Autodesk Fusion 360 part; units mm, degrees
sketch "Sketch1" plane through (0, 0, 0) normal (0, 0, 1) x (1, 0, 0)
  line L0 (0, 0) -> (50.8, 0)
  line L1 (50.8, 0) -> (50.8, 50.8)
  line L2 (50.8, 50.8) -> (0, 50.8)
  line L3 (0, 50.8) -> (0, 0)
  dimension "d1" = 50.8
  dimension "d2" = 50.8
extrude "Extrude1" add sketch "Sketch1" along normal blind 31.75
sketch "Sketch2" plane through (50.8, 0, 0) normal (1, 0, 0) x (0, 1, 0)
  line L0 (0, 0) -> (50.8, 0)
  line L1 (50.8, 0) -> (50.8, 31.75)
  line L2 (50.8, 31.75) -> (0, 31.75)
  line L3 (0, 31.75) -> (0, 0)
  line L4 (50.8, 23.368) -> (10.16, 23.368)
  line L5 (10.16, 23.368) -> (10.16, 3.81)
  line L6 (10.16, 3.81) -> (50.8, 3.81)
  line L7 (50.8, 3.81) -> (50.8, 23.368)
  dimension "d5" = 40.64
  dimension "d6" = 19.558
  dimension "d14" = 3.81
extrude "Extrude2" cut sketch "Sketch2" against normal blind 40.64 contours L1 L4 L5 L6 L7
sketch "Sketch3" plane through (0, 0, 31.75) normal (0, 0, 1) x (-1, 0, 0)
  line L0 (0, -50.8) -> (0, 0)
  line L1 (0, 0) -> (-50.8, 0)
  line L2 (-50.8, 0) -> (-50.8, -50.8)
  line L3 (-50.8, -50.8) -> (0, -50.8)
  line L4 (0, 0) -> (-25.4, 0)
  line L5 (-25.4, 0) -> (-25.4, -25.4)
  line L6 (-25.4, -25.4) -> (0, -25.4)
  line L7 (0, -25.4) -> (0, 0)
  dimension "d10" = 25.4
  dimension "d11" = 25.4
extrude "Extrude3" add sketch "Sketch3" along normal blind 152.4 contours L0 L1 L4 L5 L6 L7
fillet "Fillet1" radius 2.54 2 edges at (25.4, 12.7, 31.75) (12.7, 25.4, 31.75)
sketch "Sketch4" plane through (0, 0, 0) normal (0, 0, -1) x (1, 0, 0)
  line L0 (0, 0) -> (0, -50.8)
  line L1 (0, -50.8) -> (50.8, -50.8)
  line L2 (50.8, -50.8) -> (50.8, 0)
  line L3 (50.8, 0) -> (0, 0)
  line L4 (2.54, -2.54) -> (22.86, -2.54)
  line L5 (22.86, -2.54) -> (22.86, -22.86)
  line L6 (22.86, -22.86) -> (2.54, -22.86)
  line L7 (2.54, -22.86) -> (2.54, -2.54)
  dimension "d17" = 2.54
  dimension "d18" = 2.54
  dimension "d19" = 20.32
  dimension "d20" = 20.32
sketch "Sketch5" plane through (0, 0, 0) normal (0, 0, -1) x (1, 0, 0)
  line L0 (5.08, -5.08) -> (20.32, -5.08)
  line L1 (20.32, -5.08) -> (20.32, -20.32)
  line L2 (20.32, -20.32) -> (5.08, -20.32)
  line L3 (5.08, -20.32) -> (5.08, -5.08)
  line L4 (2.54, -2.54) -> (22.86, -2.54)
  line L5 (2.54, -22.86) -> (2.54, -2.54)
  dimension "d21" = 2.54
  dimension "d22" = 2.54
  dimension "d23" = 15.24
  dimension "d24" = 15.24
extrude "Extrude4" add sketch "Sketch5" along normal blind 2.54
loft "Loft1" add profiles "Sketch4" section 1 contours L4 L5 L6 L7 section 2 face at (10.16, 15.24, -2.54)
sketch "Sketch6" plane through (0, 0, 184.15) normal (0, 0, 1) x (-1, 0, 0)
  line L0 (0, -25.4) -> (0, 0)
  line L1 (0, 0) -> (-25.4, 0)
  line L2 (-25.4, 0) -> (-25.4, -25.4)
  line L3 (-25.4, -25.4) -> (0, -25.4)
  line L4 (-2.54, -22.86) -> (-22.86, -22.86)
  line L5 (-22.86, -22.86) -> (-22.86, -2.54)
  line L6 (-22.86, -2.54) -> (-2.54, -2.54)
  line L7 (-2.54, -2.54) -> (-2.54, -22.86)
  line L8 (-5.08, -20.32) -> (-20.32, -20.32)
  line L9 (-20.32, -20.32) -> (-20.32, -5.08)
  line L10 (-20.32, -5.08) -> (-5.08, -5.08)
  line L11 (-5.08, -5.08) -> (-5.08, -20.32)
  dimension "d27" = 2.54
  dimension "d28" = 2.54
  dimension "d29" = 2.54
  dimension "d30" = 20.32
  dimension "d31" = 2.54
  dimension "d32" = 15.24
  dimension "d33" = 15.24
  dimension "d34" = 2.54
extrude "Extrude5" cut sketch "Sketch6" against normal blind 2.54 contours L8 L9 L10 L11
loft "Loft2" cut profiles "Sketch6" section 1 contours L4 L5 L6 L7 section 2 face at (15.24, 15.24, 181.61)
Geometry: final body of the model. Coordinates: model frame, mm. A direction names the side the tool comes from. Round coordinates to 2 decimals unless told otherwise and drop trailing zeros. Order: outer loops, then holes, each group sorted by start corner. A loop starts at its lowest first (then second) coordinate and runs counter-clockwise, first axis right, second up. Notation, with made-up numbers: (38, 62) - (52, 62) arc R18 cw to (52, 84) - close; hole circle Ø7 at (88, 62.25). An arc over 180 degrees is marked (long way). Write item = value, one per line. Start each with the question number.
Q1. Cut plane A-A on y = 40.5. Return the cut outline in (x, z), and give its area (3 significant figures).
Q2. Pull-direction query (Y, two-part tool) for faces 1 (the flat face through (31, 31, 23.368)), 2 (the flat face through (13, 13, 181.61)), 3 (the flat face through (20, 50.8, 26)); classes: +Y half, -Y half, draft (parallel to the pull), parting line (faces both ways), or undercut.
Q3. Pin query (flat end, axial travel): pin 1 (3 mm diameter, centred on x = 29.5, y = 9.5, fed in from +Z); pin 2 (7.5 mm diameter, centred on x = 9, y = 14.5, fed in from +Z); pin 3 (6 mm diameter, centred on x = 24, z = 18.5, fed in from +Y). Return the tip coordinate at first contact, or that it passes through.
Q4. Ray query, line 1 (Z direction, x = 28, y = 31); line 2 (X direction, y = 25, z = 108). Return the intervals inside material, ascending. Write a range as from..to.
Q5. Cut plane C-C on z = 133. Return the cut outline in (x, y).
Q6. Access query for faces 4 (the flat face through (10.16, 30, 14)), 5 (the flat face through (31, 31, 31.75)), 6 (the flat face through (13, 25.4, 108)). Directions: +Z, -Z, +X, -X, +Y, -Y. A direction counts if a zero-diameter tool reaches every point of the face in a straight line with its end or side. Return the directions, or none.
Outcome:
q1.outline = (0, 0) - (50.8, 0) - (50.8, 3.81) - (10.16, 3.81) - (10.16, 23.37) - (50.8, 23.37) - (50.8, 31.75) - (0, 31.75) - close
q1.area = 818 mm^2
q2.face_1 = draft
q2.face_2 = undercut
q2.face_3 = +Y half
q3.pin_1 = 31.75
q3.pin_2 = 181.61
q3.pin_3 = 10.16
q4.line_1 = 0..3.81, 23.37..31.75
q4.line_2 = 0..25.4
q5.outline = (0, 0) - (25.4, 0) - (25.4, 25.4) - (0, 25.4) - close
q6.face_4 = +X, +Y
q6.face_5 = +Z, +X, +Y
q6.face_6 = +Z, +X, -X, +Y
